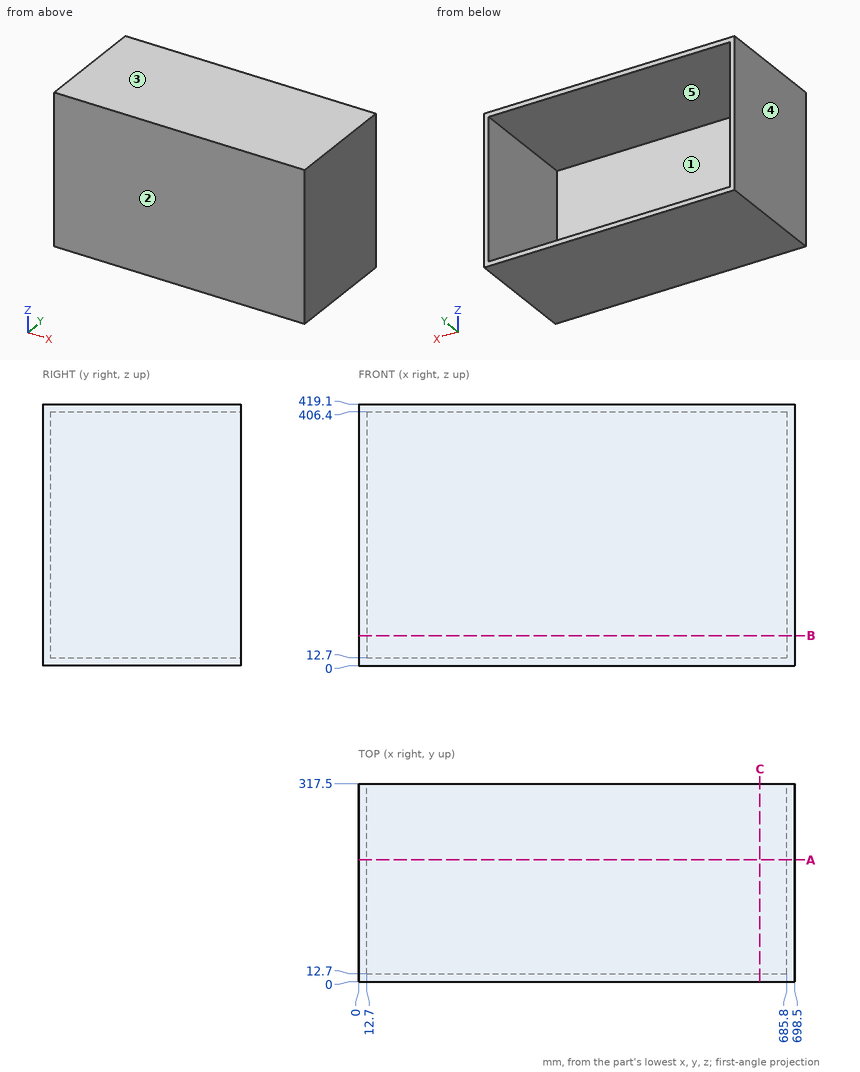
The figure shows three views and two pictorial views of one solid part (mm, origin at its lowest corner). Answer the questions. A direction names the side the tool comes from. Coordinates: 2 decimals unless noted, no trailing zeros. Loops run counter-clockwise (first coordinate to the right, second up) from the corner with the lowest first, then second, coordinate; pieces in that order, holes last.
(1) The part is cut by section B-B (z = 48). Determine the outline of the cut face in (x, y).
Solution:
outline: (0, 0) - (698.5, 0) - (698.5, 317.5) - (685.8, 317.5) - (685.8, 12.7) - (12.7, 12.7) - (12.7, 317.5) - (0, 317.5) - close
(2) Consider line 1 along Z through (x, y) = (629, 110); line 2 along X through (y, z) = (227, 291.5); line 3 along Y through (x, z) = (238, 188.5). Determine where each line is inside the solid, lowest interval first.
Solution:
line 1: z = 0 to 12.7, 406.4 to 419.1
line 2: x = 0 to 12.7, 685.8 to 698.5
line 3: y = 0 to 12.7
(3) The part is cut by section A-A (y = 195). Determine the outline of the cut face in (x, z).
Solution:
outline: (0, 0) - (698.5, 0) - (698.5, 419.1) - (0, 419.1) - close; hole (12.7, 12.7) - (685.8, 12.7) - (685.8, 406.4) - (12.7, 406.4) - close
(4) The mould has two halves that part along Z. Classify the marked faces 3, 4 and 5: released by +Z, released by -Z, zero draft, split by the parting line, or undercut.
Solution:
face 3: released by +Z
face 4: zero draft
face 5: undercut
(5) A flat-ended cylindrical pin translates along its axis: pin 1 Ø1.5 at (x, z) = (571.5, 234) entering from +Y. Find the tip coordinate at first contact, or state that the pin passes through.
Solution:
pin 1: stops at y = 12.7
(6) A tool of negligible diameter and unlimited length cuts with its end or side. For the marked faces 1 and 2, from which of +Z, -Z, +X, -X, +Y, -Y can it reach the whole face along a straight path? Write none if from no direction.
Solution:
face 1: +Y
face 2: +Z, -Z, +X, -X, -Y
(7) The part is cut by section C-C (x = 643). Determine the outline of the cut face in (y, z).
Solution:
outline: (0, 0) - (317.5, 0) - (317.5, 12.7) - (12.7, 12.7) - (12.7, 406.4) - (317.5, 406.4) - (317.5, 419.1) - (0, 419.1) - close
